from build123d import *

# Parameters (mm, degrees)
SKETCH1_W                        = 254
SKETCH1_H                        = 44.45
BOSS_EXTRUDE1_DEPTH              = 3.175
FILLET1_R                        = 6.35
F_17_64_0_26563_DIAMETER_HOLE1_D = 6.747002


with BuildPart() as part:
    # Sketch1 → Boss-Extrude1 (new body)
    with BuildSketch(Plane(origin=(0, 0, 0), x_dir=(1, 0, 0), z_dir=(0, 1, 0))):
        with Locations((127, 22.225)):
            Rectangle(SKETCH1_W, SKETCH1_H)
    extrude(amount=BOSS_EXTRUDE1_DEPTH)

    # Fillet1
    fillet1_edges = [part.edges().sort_by_distance(p)[0] for p in [
        (0, 1.5875, -44.45),
        (254, 1.5875, -44.45),
        (254, 1.5875, 0),
        (0, 1.5875, 0),
    ]]
    fillet(fillet1_edges, radius=FILLET1_R)

    # 17/64 (0.26563) Diameter Hole1 (through all)
    with Locations(Plane(origin=(0, 3.175, 0), x_dir=(1, 0, 0), z_dir=(0, 1, 0))):
        with Locations((12.7, 34.925), (241.3, 34.925)):
            Hole(F_17_64_0_26563_DIAMETER_HOLE1_D / 2)


solid = part.part
Build history of the part. All positions in model axes, mm. Coordinates: 2 decimals unless noted, no trailing zeros. One line per question, with ' | ' between items. Start each with the question number.
Q1. Probe L1, parallel to X at y = 2.8, z = -35.5; L2, parallel to Z at x = 241.3, y = 1.4; L3, parallel to X at y = 2.35, z = -35. List the from-to ranges inside material, lowest first. Write a range as from..to.
Q2. Two-plate mould, pull along Z, no slides. Class faces 1 (the face through (1.81, 1.61, -42.54)), 2 (the face through (252.09, 1.61, -1.81)), 3 (the face through (238.082, 1.565, -35.938)), 4 (the face through (10.89, 1.57, -37.77)): +Z half, -Z half, draft (parallel to the pull), parting line (faces both ways), or undercut.
Q3. Flat gauge pin, fed straight in: pin 1 Ø5.5 at (x, z) = (12.7, -34.925) entering from +Y. Where does the tip first touch, or does it go through?
Check values:
1) L1: x = 0..9.38, 16.02..237.98, 244.62..254 | L2: z = -44.45..-38.3, -31.55..0 | L3: x = 0..9.33, 16.07..237.93, 244.67..254
2) face 1: -Z half | face 2: +Z half | face 3: undercut | face 4: undercut
3) pin 1: passes through
